Answer from the drawing. Dimensions are ordinates in mm from the lowest x, y and z of the part. A direction names the side the tool comes from. Give positions to 0.01 mm unless a question says otherwise; leave off trailing zeros. Loops run counter-clockwise (first coordinate to the right, second up) from the corner with the lowest first, then second, coordinate; pieces in that order, holes last. Notation, with made-up numbers: (58.25, 16) - (81.25, 16) arc R4 cw to (81.25, 21) - close; hole circle Ø10 at (43, -27). An arc over 180 degrees is marked (long way). One line per item, written item: value.
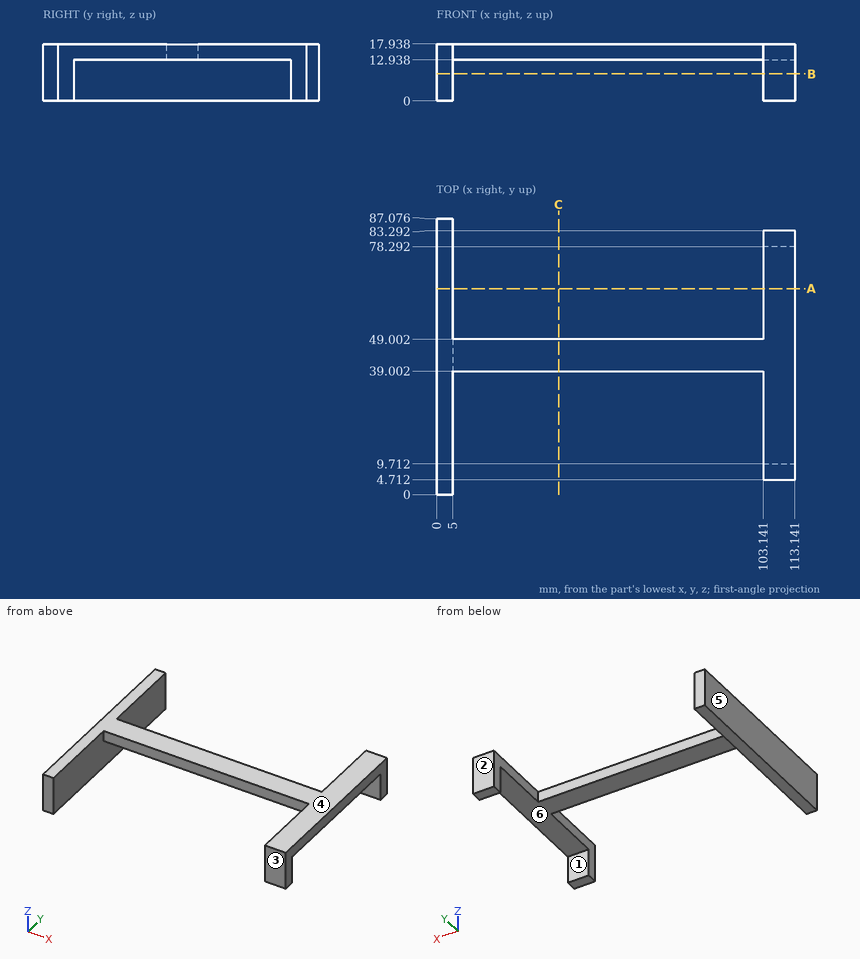
1. For the marked faces 5 and 6, determine the directions among +Z, -Z, +X, -X, +Y, -Y from which every point of the face is accessible in a straight line to the end or side of a thin tool.
Output:
face 5: +Z, -Z, -X, +Y, -Y
face 6: -Z, +X
2. The mould has two halves that part along Y. Classify the marked faces 1, 2, 3 and 4: released by +Y, released by -Y, zero draft, split by the parting line, or undercut.
Output:
face 1: undercut
face 2: released by +Y
face 3: released by -Y
face 4: zero draft
3. Section A-A (y = 65) is taken. Write down the section's boundary in (x, z).
Output:
outline: (0, 0) - (5, 0) - (5, 17.94) - (0, 17.94) - close; (103.14, 12.94) - (113.14, 12.94) - (113.14, 17.94) - (103.14, 17.94) - close
4. Section C-C (x = 38.5) is taken. Write down the section's boundary in (y, z), and give its area (3 significant figures).
Output:
outline: (39, 12.94) - (49, 12.94) - (49, 17.94) - (39, 17.94) - close
area: 50.0 mm²
5. Flat-ended cylindrical pins translate along their axes: pin 1 Ø3 at (x, z) = (109, 11.5) entering from -Y; pin 2 Ø6 at (y, z) = (29, 8) entering from +X; pin 3 Ø4 at (x, z) = (85.5, 13.5) entering from +Y. Find the tip coordinate at first contact, or state that the pin passes through.
Output:
pin 1: stops at y = 4.71
pin 2: stops at x = 5
pin 3: stops at y = 49
6. Section B-B (z = 8.5) is taken. Write down the section's boundary in (x, y) (1 decimal).
Output:
outline: (0, 0) - (5, 0) - (5, 87.1) - (0, 87.1) - close; (103.1, 4.7) - (113.1, 4.7) - (113.1, 9.7) - (103.1, 9.7) - close; (103.1, 78.3) - (113.1, 78.3) - (113.1, 83.3) - (103.1, 83.3) - close
7. Find the intervals of material crossed by line 1 along X through (y, z) = (75.5, 17); line 2 along Y through (x, z) = (105, 12); line 3 along X through (y, z) = (54, 8), in increasing order.
Output:
line 1: x = 0 to 5, 103.14 to 113.14
line 2: y = 4.71 to 9.71, 78.29 to 83.29
line 3: x = 0 to 5
